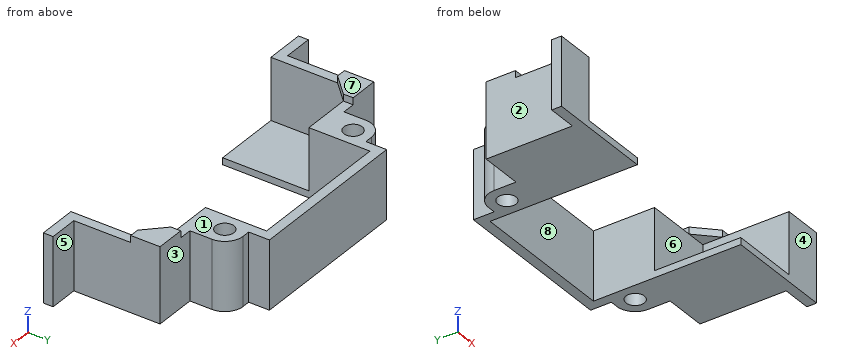
Autodesk Inventor part; units mm, degrees
ref_plane "YZ Plane" through (0, 0, 0) normal (1, 0, 0) x (0, 1, 0)
ref_plane "XZ Plane" through (0, 0, 0) normal (0, 1, 0) x (-1, 0, 0)
ref_plane "XY Plane" through (0, 0, 0) normal (0, 0, 1) x (1, 0, 0)
sketch "スケッチ1" plane through (0, 0, 0) normal (0, 0, 1) x (1, 0, 0)
  line L0 (0, 0) -> (0, 17.65)
  line L1 (0, 17.65) -> (28, 17.65)
  line L2 (28, 17.65) -> (28, 30.15)
  line L3 (28, 30.15) -> (58, 30.15)
  line L4 (58, 30.15) -> (58, 0)
  line L5 (58, 0) -> (60, 0)
  line L6 (60, 0) -> (60, 32.15)
  line L7 (60, 32.15) -> (28, 32.15)
  line L8 (28, 32.15) -> (26, 32.15)
  line L9 (26, 32.15) -> (26, 19.65)
  line L10 (26, 19.65) -> (-2, 19.65)
  line L11 (-2, 19.65) -> (-2, 0)
  line L12 (-2, 0) -> (0, 0)
  dimension "d0" = 17.65
  dimension "d1" = 28
  dimension "d2" = 12.5
  dimension "d3" = 30
  dimension "d4" = 2
  dimension "d5" = 32.15
  dimension "d6" = 32
  dimension "d7" = 2
  dimension "d8" = 12.5
  dimension "d9" = 28
extrude "押し出し1" add sketch "スケッチ1" along normal blind 14
sketch "スケッチ2" plane through (60, 0, 0) normal (1, 0, 0) x (0, 0, -1)
  line L0 (0, 0) -> (-14, 0)
  line L1 (-14, 0) -> (0, 0)
  line L2 (0, 0) -> (0, 2)
  line L3 (0, 2) -> (-14, 2)
  line L4 (-14, 2) -> (-14, 0)
  dimension "d12" = 14
  dimension "d13" = 2
extrude "押し出し2" add sketch "スケッチ2" along normal blind 7
sketch "スケッチ3" plane through (-2, 0, 0) normal (-1, 0, 0) x (0, 0, 1)
  line L0 (14, 2) -> (0, 2)
  line L1 (0, 0) -> (14, 0)
  line L2 (14, 0) -> (14, 2)
  line L3 (14, 2) -> (0, 2)
  line L4 (0, 2) -> (0, 0)
  dimension "d16" = 14
extrude "押し出し3" add sketch "スケッチ3" along normal blind 7
sketch "スケッチ4" plane through (0, 0, 14) normal (0, 0, 1) x (1, 0, 0)
  line L0 (60, 32.15) -> (60, 24.15)
  line L1 (60, 24.15) -> (61.6, 24.15)
  arc A0 (61.6, 20.4) -> (61.6, 27.9) centre (61.6, 24.15) ccw
  line L2 (61.6, 24.15) -> (61.6, 20.4) construction
  line L3 (61.6, 24.15) -> (61.6, 27.9) construction
  line L4 (61.6, 27.9) -> (60, 27.9)
  line L5 (61.6, 20.4) -> (60, 20.4)
  line L6 (60, 2) -> (60, 32.15)
  line L7 (60, 27.9) -> (60, 20.4)
  point P0 (0, 0)
  dimension "d47" = 8
  dimension "d48" = 1.6
  dimension "d49" = 3.75
  dimension "d50" = 180
extrude "押し出し4" add sketch "スケッチ4" against normal blind 14
hole "穴3" at (61.6, 24.15, 14) direction (0, 0, -1) diameter 3.75 end through all
sketch "スケッチ7" plane through (0, 0, 14) normal (0, 0, 1) x (1, 0, 0)
  line L0 (60, 32.15) -> (26, 32.15)
  line L1 (26, 32.15) -> (26, 24.15)
  line L2 (26, 24.15) -> (24.4, 24.15)
  arc A0 (24.4, 27.9) -> (24.4, 20.4) centre (24.4, 24.15) ccw
  line L3 (24.4, 27.9) -> (26, 27.9)
  line L4 (24.4, 20.4) -> (26, 20.4)
  line L5 (26, 20.4) -> (26, 27.9)
  line L6 (26, 32.15) -> (26, 19.65)
  circle A1 centre (24.4, 24.15) radius 1.875
  point P0 (0, 0)
  dimension "d60" = 8
  dimension "d61" = 1.6
  dimension "d62" = 3.75
  dimension "d63" = 3.75
extrude "押し出し6" add sketch "スケッチ7" against normal blind 14 contours L1 A1 L5 L4 A0 L3 | L1 L5 A1 picked at (23.6929, 24.15)
hole "穴4" at (24.4, 24.15, 14) direction (0, 0, -1) diameter 3.75 end through all
sketch "スケッチ10" plane through (0, 17.65, 0) normal (0, -1, 0) x (1, 0, 0)
  line L0 (28, 14) -> (58, 14)
  line L1 (0, 0) -> (28, 0)
  line L2 (28, 0) -> (28, 14)
  line L3 (28, 14) -> (0, 14)
  line L4 (0, 14) -> (0, 0)
extrude "押し出し7" cut sketch "スケッチ10" against normal blind 0.6
sketch "スケッチ11" plane through (0, 0, 0) normal (0, -1, 0) x (1, 0, 0)
  line L0 (0, 14) -> (-9, 14)
  line L1 (60, 0) -> (67, 0)
  line L2 (-9, 14) -> (67, 14)
  line L3 (67, 14) -> (67, 0)
  line L4 (67, 0) -> (-9, 0)
  line L5 (-9, 0) -> (-9, 14)
  point P0 (0, 0)
extrude "押し出し8" cut sketch "スケッチ11" against normal blind 0.6
sketch "スケッチ12" plane through (0, 0, 14) normal (0, 0, 1) x (1, 0, 0)
  line L0 (-2, 19.65) -> (-2, 2)
  line L1 (-2, 19.65) -> (4, 19.65)
  line L2 (26, 19.65) -> (-2, 19.65)
  line L3 (4, 19.65) -> (4, 18.25)
  line L4 (0, 18.25) -> (28, 18.25)
  line L5 (4, 18.25) -> (0.2844, 14.5344)
  line L6 (4, 18.25) -> (9.2547, 18.25) construction
  line L7 (0.2844, 14.5344) -> (0, 14.25)
  line L8 (0, 0.6) -> (0, 18.25)
  line L9 (0, 14.25) -> (-2, 14.25)
  line L10 (-2, 14.25) -> (-2, 19.65)
  point P0 (0, 0)
  dimension "d79" = 6
  dimension "d80" = 135
extrude "押し出し9" add sketch "スケッチ12" along normal blind 2
sketch "スケッチ15" plane through (0, 0, 0) normal (0, 0, -1) x (-1, 0, 0)
  line L0 (0, 0.6) -> (0, 18.25)
  line L1 (0, 18.25) -> (-14, 18.25)
  line L2 (-14, 18.25) -> (-14, 0.6)
  line L3 (-14, 0.6) -> (0, 0.6)
  line L4 (0, 0.6) -> (0, 18.25)
  point P0 (0, 0)
  dimension "d88" = 14
extrude "押し出し11" add sketch "スケッチ15" against normal blind 1.4
sketch "スケッチ17" plane through (67, 0, 0) normal (1, 0, 0) x (0, 0, -1)
  line L0 (0, 0.6) -> (-14, 0.6)
  line L1 (0, 0.6) -> (-14, 0.6)
  line L2 (-14, 0.6) -> (-14, 9.5309)
  line L3 (-14, 9.5309) -> (0, 9.5309)
  line L4 (0, 9.5309) -> (0, 0.6)
  point P0 (0, 0)
extrude "押し出し13" cut sketch "スケッチ17" against normal blind 3
sketch "スケッチ18" plane through (-9, 0, 0) normal (-1, 0, 0) x (0, 0, 1)
  line L0 (0, 0.6) -> (14, 0.6)
  line L1 (0, 0.6) -> (14, 0.6)
  line L2 (14, 0.6) -> (14, 6.5)
  line L3 (14, 6.5) -> (0, 6.5)
  line L4 (0, 6.5) -> (0, 0.6)
  point P0 (0, 0)
extrude "押し出し14" cut sketch "スケッチ18" against normal blind 3
hole "穴5" at (-4, 2, 7) direction (0, -1, 0) diameter 2.4 end through all
hole "穴6" at (62, 2, 7) direction (0, -1, 0) diameter 2.4 end through all
mirror "ミラー1" about plane through (31.8158, 20.0509, 0) normal (0, 0, -1) of "押し出し3", "押し出し1", "押し出し4", "穴3", "押し出し2", "穴6", "穴4", "押し出し6", "押し出し7", "押し出し9", "押し出し11", "押し出し14", "押し出し13", "穴5", "押し出し8"
sketch "スケッチ19" plane through (0, 0, 14) normal (0, 0, 1) x (1, 0, 0)
  line L0 (94.8832, 81.412) -> (-62.365, 81.412)
  line L1 (-62.365, 81.412) -> (-62.365, -71.7744)
  line L2 (-62.365, -71.7744) -> (94.8832, -71.7744)
  line L3 (94.8832, -71.7744) -> (94.8832, 81.412)
  point P0 (0, 0)
extrude "押し出し15" cut sketch "スケッチ19" against normal blind 14
sketch "スケッチ20" plane through (-2, 19.65, 14) normal (0, 1, 0) x (1, 0, 0)
  line L0 (17.6833, -4.2941) -> (-12.6138, -4.2941)
  line L1 (-12.6138, -4.2941) -> (-12.6138, 1.0873)
  line L2 (-12.6138, 1.0873) -> (17.6833, 1.0873)
  line L3 (17.6833, 1.0873) -> (17.6833, -4.2941)
  point P0 (2, 14)
extrude "押し出し16" cut sketch "スケッチ20" against normal blind 14
sketch "スケッチ21" plane through (26, 27.9, -14) normal (-1, 0, 0) x (0, 0, 1)
  line L0 (0, -8.25) -> (-2, -8.25)
  line L1 (-2, -8.25) -> (18.9234, -8.25)
  line L2 (18.9234, -8.25) -> (18.9234, 5.2405)
  line L3 (18.9234, 5.2405) -> (-2, 5.2405)
  line L4 (-2, 5.2405) -> (-2, -8.25)
  point P0 (14, -27.9)
split body "分割1" sketch "スケッチ21" result one side removed curves L2 L3 L4 L1 removed pieces at (9.3333, 19.15, -4.6667) (58.5, 13.3, -4.6667)
sketch "スケッチ22" plane through (0, 0, 0) normal (0, 0, 1) x (1, 0, 0)
  line L0 (28, 19.65) -> (28, 30.15)
  line L1 (28, 19.65) -> (28, 17.65)
  line L2 (28, 17.65) -> (14, 17.65)
  line L3 (14, 17.65) -> (14, 0)
  line L4 (14, 17.65) -> (31.65, 17.65) construction
  line L5 (14, 0) -> (8, 0)
  line L6 (8, 0) -> (8, 2)
  line L7 (8, 2) -> (12, 2)
  line L8 (26.0798, 19.65) -> (12, 19.65)
  line L9 (12, 19.65) -> (12, 2)
  line L10 (58, 19.65) -> (60, 19.65)
  line L11 (58, 19.65) -> (58, 17.65)
  line L12 (58, 17.65) -> (72, 17.65)
  line L13 (72, 17.65) -> (72, 0)
  line L14 (72, 0) -> (78, 0)
  line L15 (78, 0) -> (78, 2)
  line L16 (78, 2) -> (74, 2)
  line L17 (74, 2) -> (74, 19.65)
  line L18 (74, 19.65) -> (60, 19.65)
  line L19 (26.0798, 19.65) -> (28, 19.65)
  line L20 (24.4, 20.4) -> (26, 20.4)
  line L21 (58, 19.65) -> (60, 19.65)
  point P0 (0, 0)
  dimension "d119" = 2
  dimension "d120" = 14
  dimension "d121" = 17.65
  dimension "d122" = 90
  dimension "d123" = 6
  dimension "d124" = 2
  dimension "d125" = 4
  dimension "d126" = 14
  dimension "d127" = 6
  dimension "d128" = 2
  dimension "d129" = 4
extrude "押し出し17" add sketch "スケッチ22" against normal blind 14
sketch "スケッチ23" plane through (26, 32.15, -14) normal (0, 1, 0) x (1, 0, 0)
  line L0 (32, -14) -> (2, -14)
  line L1 (17, -14) -> (17, 0)
  line L2 (2, 0) -> (32, 0)
  point P0 (-26, -14)
sketch "スケッチ25" plane through (24.4, 24.15, -14) normal (0, 0, -1) x (-1, 0, 0)
  line L0 (-3.6, -6.5) -> (10.4, -6.5)
  line L1 (10.4, -6.5) -> (-3.6, -6.5)
  line L2 (-3.6, -6.5) -> (-3.6, -24.15)
  line L3 (-3.6, -24.15) -> (10.4, -24.15)
  line L4 (10.4, -24.15) -> (10.4, -6.5)
  point P0 (24.4, -24.15)
extrude "押し出し18" add sketch "スケッチ25" against normal blind 1.4
ref_plane "作業平面1" through (43, 32.15, 0) normal (1, 0, 0) x (0, 0, -1)
mirror "ミラー3" about plane through (43, 32.15, 0) normal (1, 0, 0) of "押し出し18"
sketch "スケッチ26" plane through (0, 0, 0) normal (0, 0, 1) x (1, 0, 0)
  line L0 (12, 2) -> (12, 19.65)
  line L1 (12, 19.65) -> (18, 19.65)
  line L2 (12, 19.65) -> (26, 19.65)
  line L3 (18, 19.65) -> (18, 17.65)
  line L4 (28, 17.65) -> (14, 17.65)
  line L5 (18, 17.65) -> (14, 13.65)
  line L6 (14, 17.65) -> (14, 0)
  line L7 (18, 17.65) -> (23.6569, 17.65) construction
  line L8 (14, 13.65) -> (12, 13.65)
  line L9 (12, 13.65) -> (12, 19.65)
  point P0 (0, 0)
  dimension "d139" = 6
  dimension "d140" = 135
extrude "押し出し20" add sketch "スケッチ26" along normal blind 1.4
mirror "ミラー4" about plane through (43, 32.15, 0) normal (1, 0, 0) of "押し出し20"
sketch "スケッチ27" plane through (0, 0, 0) normal (0, 0, 1) x (1, 0, 0)
  line L0 (8, 2) -> (12, 2)
  line L1 (8, 2) -> (6, 2)
  line L2 (6, 2) -> (6, 0)
  line L3 (6, 0) -> (8, 0)
  line L4 (8, 0) -> (8, 2)
  line L5 (78, 2) -> (80, 2)
  line L6 (80, 2) -> (80, 0)
  line L7 (80, 0) -> (78, 0)
  line L8 (78, 0) -> (78, 2)
  point P0 (0, 0)
  dimension "d143" = 2
  dimension "d144" = 2
extrude "押し出し21" add sketch "スケッチ27" against normal blind 14
hole "穴7" at (77, 2, -7) direction (0, -1, 0) diameter 2.4 end through all
hole "穴8" at (9, 2, -7) direction (0, -1, 0) diameter 2.4 end through all
sketch "スケッチ28" plane through (0, 0, 0) normal (0, 0, 1) x (1, 0, 0)
  arc A0 (24.4, 27.9) -> (24.4, 20.4) centre (24.4, 24.15) ccw
  line L0 (20.65, 24.15) -> (20.65, 19.65)
  line L1 (12, 19.65) -> (26, 19.65)
  line L2 (24.4, 20.4) -> (26, 20.4)
  line L3 (26, 19.65) -> (26, 20.4)
  line L4 (26, 20.4) -> (20.65, 24.15)
  point P0 (0, 0)
extrude "押し出し22" add sketch "スケッチ28" against normal blind 14 contours A0 L2 L3 L1 L0
mirror "ミラー5" about plane through (43, 32.15, 0) normal (1, 0, 0) of "押し出し22"
sketch "スケッチ29" plane through (74, 2, 0) normal (0, 1, 0) x (1, 0, 0)
  circle A0 centre (3, 7) radius 1.2
  circle A1 centre (3, 7) radius 1.2
  circle A2 centre (-65, 7) radius 1.2
  circle A3 centre (-65, 7) radius 1.2
  point P0 (-74, 0)
extrude "押し出し23" add sketch "スケッチ29" against normal blind 2
properties part number "センサ冶具1セット穴埋めver"
Part model, mm, in its own coordinate system. Face numbers are marked on the shaded views. A direction names the side the tool comes from. Coordinates: 2 decimals unless noted, no trailing zeros. Order: outer loops, then holes, each group sorted by start corner. A loop starts at its lowest first (then second) coordinate and runs counter-clockwise, first axis right, second up. Notation, with made-up numbers: M 3,57 L 61,57 A7 ccw 61,69 Z; hole C -19,10.25 d5. An arc over 180 degrees is marked long. Use a Markdown table: item, result.
(1) Flat gauge pins, fed straight in: pin 1 (2 mm diameter, centred on y = 23.5, z = -5, fed in from +X); pin 2 (1.5 mm diameter, centred on x = 15, z = -2, fed in from -Y); pin 3 (4.5 mm diameter, centred on x = 61.6, y = 24.15, fed in from +Z). Where does each tip first touch, or does it go through?
A:
| item | result |
|---|---|
| pin 1 | stops at x = 65.35 |
| pin 2 | stops at y = 17.65 |
| pin 3 | stops at z = 0 |
(2) Cut at B-B on z = -11. Write the cut outline in (x, y) (3 decimals).
A:
| item | result |
|---|---|
| outline | M 6,0 L 14,0 L 14,17.65 L 28,17.65 L 28,30.15 L 58,30.15 L 58,17.65 L 72,17.65 L 72,0 L 80,0 L 80,2 L 74,2 L 74,19.65 L 65.35,19.65 L 65.35,24.15 A3.75 ccw 61.6,27.9 L 60,27.9 L 60,32.15 L 26,32.15 L 26,27.9 L 24.4,27.9 A3.75 ccw 20.65,24.15 L 20.65,19.65 L 12,19.65 L 12,2 L 6,2 Z; hole C 24.4,24.15 d3.75; hole C 61.6,24.15 d3.75 |
(3) Probe L1, parallel to X at y = 24.15, z = -9 (3 decimals); L2, parallel to Y at x = 24.4, z = -4.5 (3 decimals); L3, parallel to X at y = 7.5, z = -4. List the from-to ranges inside material, lowest first.
A:
| item | result |
|---|---|
| L1 | x = 20.65 to 22.525, 26.275 to 28, 58 to 59.725, 63.475 to 65.35 |
| L2 | y = 17.65 to 22.275, 26.025 to 27.9 |
| L3 | x = 12 to 14, 72 to 74 |
(4) Cut at A-A on y = 14.5. Write the cut outline in (x, z).
A:
| item | result |
|---|---|
| outline | M 12,-14 L 28,-14 L 28,-12.6 L 14,-12.6 L 14,0 L 14.85,0 L 14.85,1.4 L 12,1.4 Z; M 58,-14 L 74,-14 L 74,1.4 L 71.15,1.4 L 71.15,0 L 72,0 L 72,-12.6 L 58,-12.6 Z |
(5) Cut at D-D on y = 25. Write the cut outline in (x, z), then the cut area to 3 significant figures.
A:
| item | result |
|---|---|
| outline | M 20.75,-14 L 22.73,-14 L 22.73,0 L 20.75,0 Z; M 26.07,-14 L 28,-14 L 28,0 L 26.07,0 Z; M 58,-14 L 59.93,-14 L 59.93,0 L 58,0 Z; M 63.27,-14 L 65.25,-14 L 65.25,0 L 63.27,0 Z |
| area | 109 mm^2 |
(6) Pull direction X, two halves, no side cores. Call the marked faces 1, 2 and 3: released by +X, released by -X, zero draft, split by the parting line, or undercut.
A:
| item | result |
|---|---|
| face 1 | undercut |
| face 2 | released by -X |
| face 3 | zero draft |
(7) Cut at C-C on x = 16.5. Write the cut outline in (y, z), then the cut area to 3 significant figures.
A:
| item | result |
|---|---|
| outline | M 0,-14 L 19.65,-14 L 19.65,1.4 L 16.15,1.4 L 16.15,0 L 17.65,0 L 17.65,-12.6 L 0,-12.6 Z |
| area | 57.6 mm^2 |
(8) Tool access for the marked faces 4, 5, 6, 7 and 8: list every direction of +Z, -Z, +X, -X, +Y, -Y with a clear straight run to the whole face (end or side of a thin tool).
A:
| item | result |
|---|---|
| face 4 | +Z, -Z, +X, -X, -Y |
| face 5 | +Z, -Z, +X, +Y |
| face 6 | -Y |
| face 7 | +Z, +X, -X, +Y, -Y |
| face 8 | +Z, -Z, -Y |
